Job drawing, mm, ordinate dimensions from the low corner. One solid piece. A direction names the side the tool comes from. Give positions to 0.01 mm unless a question says otherwise; leave off trailing zeros. Loops run counter-clockwise (first coordinate to the right, second up) from the corner with the lowest first, then second, coordinate; pieces in that order, holes last.
Item 1: Saw through at C-C on z = 1.8. Give the cut face in (x, y), plus the area to 3 significant figures.
Item 2: Which spindle directions (+Z, -Z, +X, -X, +Y, -Y) get a long thin tool onto all of the face, cutting with end or side? Do the marked faces 1 and 2. Say none if no direction does.
Item 3: Mould opens along X. For the marked faces 3, 4, 5 and 6 say: released by +X, released by -X, zero draft, split by the parting line, or undercut.
Item 4: Saw through at A-A on x = 12. Give the cut face in (y, z), plus the area to 3 significant figures.
Item 5: Drop flat-ended pins along their axis: P1, Ø1.9, axis at x = 16, y = 13, coming from the -Z side; P2, Ø2, axis at x = 16.71, y = 12.6, coming from the +Z side. Give the stop position or say it passes through.
Item 6: Probe probe 1 along X at (y, z) = (14.5, 0.75); probe 2 along X at (y, z) = (11.5, 1.35) (1 decimal); probe 3 along Y at (x, z) = (12, 2.1). List the from-to ranges inside material, lowest first.
Item 7: Saw through at D-D on y = 11. Give the cut face in (x, z).
Item 8: Saw through at B-B on y = 2.25. Give the cut face in (x, z).
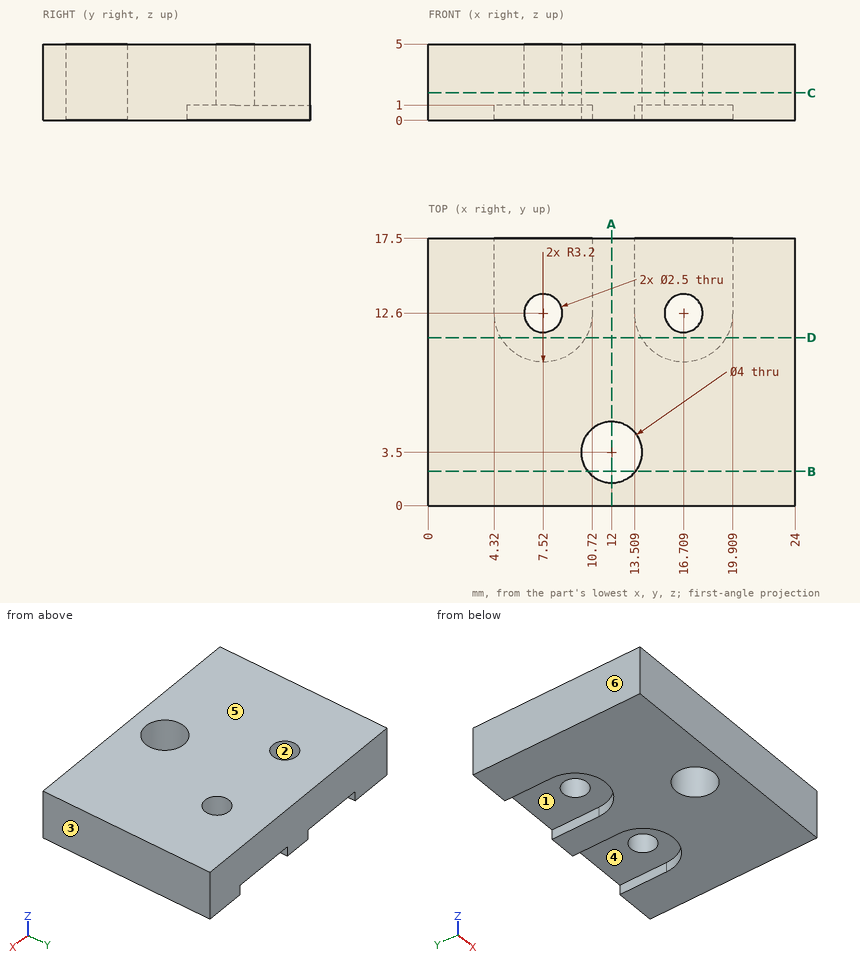
Results below:
1. outline: (0, 0) - (24, 0) - (24, 17.5) - (0, 17.5) - close; hole circle Ø2.5 at (7.52, 12.6); hole circle Ø4 at (12, 3.5); hole circle Ø2.5 at (16.71, 12.6)
1. area: 398 mm2
2. face 1: -Z, +Y
2. face 2: +Z, -Z
3. face 3: released by +X
3. face 4: undercut
3. face 5: zero draft
3. face 6: released by -X
4. outline: (0, 0) - (1.5, 0) - (1.5, 5) - (0, 5) - close; (5.5, 0) - (17.5, 0) - (17.5, 5) - (5.5, 5) - close
4. area: 67.5 mm2
5. P1: stops at z = 1
5. P2: passes through
6. probe 1: x = 0 to 4.32, 10.72 to 13.51, 19.91 to 24
6. probe 2: x = 0 to 6.9, 8.1 to 16.1, 17.3 to 24
6. probe 3: y = 0 to 1.5, 5.5 to 17.5
7. outline: (0, 0) - (4.75, 0) - (4.75, 1) - (10.29, 1) - (10.29, 0) - (13.94, 0) - (13.94, 1) - (19.48, 1) - (19.48, 0) - (24, 0) - (24, 5) - (0, 5) - close
8. outline: (0, 0) - (10.44, 0) - (10.44, 5) - (0, 5) - close; (13.56, 0) - (24, 0) - (24, 5) - (13.56, 5) - close
